```python
from build123d import *

# Parameters (mm, degrees)
ESQUISSE1_W                                    = 32
ESQUISSE1_H                                    = 18
BOSS_EXTRU_1_DEPTH                             = 2
ESQUISSE2_W                                    = 19
ESQUISSE2_H                                    = 14
BOSS_EXTRU_2_DEPTH                             = 1.4
FRAISAGE_POUR_VIS_T_TE_FRAIS_E_M21_D           = 2.6
FRAISAGE_POUR_VIS_T_TE_FRAIS_E_M21_CSINK_D     = 4.4
FRAISAGE_POUR_VIS_T_TE_FRAIS_E_M21_CSINK_ANGLE = 90
ESQUISSE6_W                                    = 15.8
ESQUISSE6_H                                    = 2
BOSS_EXTRU_3_DEPTH                             = 1.4
ESQUISSE7_W                                    = 19.2
ESQUISSE7_H                                    = 1.2
BOSS_EXTRU_4_DEPTH                             = 3.4
CONG_7_R                                       = 1


with BuildPart() as part:
    # Esquisse1 → Boss.-Extru.1 (new body)
    with BuildSketch(Plane.XY):
        Rectangle(ESQUISSE1_W, ESQUISSE1_H)
    extrude(amount=BOSS_EXTRU_1_DEPTH)

    # Esquisse2 → Boss.-Extru.2 (add)
    with BuildSketch(Plane(origin=(0, 0, 0), x_dir=(-1, 0, 0), z_dir=(0, 0, -1))):
        Rectangle(ESQUISSE2_W, ESQUISSE2_H)
    extrude(amount=BOSS_EXTRU_2_DEPTH)

    # Fraisage pour vis à tête fraisée M21 (through all)
    with Locations(Plane.XY.offset(2)):
        with Locations((-13, 0)):
            fraisage_pour_vis_t_te_frais_e_m21 = CounterSinkHole(FRAISAGE_POUR_VIS_T_TE_FRAIS_E_M21_D / 2, FRAISAGE_POUR_VIS_T_TE_FRAIS_E_M21_CSINK_D / 2, counter_sink_angle=FRAISAGE_POUR_VIS_T_TE_FRAIS_E_M21_CSINK_ANGLE)

    # Symétrie1: Fraisage pour vis à tête fraisée M21 across plane
    add(fraisage_pour_vis_t_te_frais_e_m21.mirror(Plane(origin=(0, 0, 0), x_dir=(0, 0, 1), z_dir=(1, 0, 0))), mode=Mode.SUBTRACT)

    # Esquisse6 → Boss.-Extru.3 (add)
    with BuildSketch(Plane(origin=(0, 0, 0), x_dir=(-1, 0, 0), z_dir=(0, 0, -1))):
        with Locations((0, 8)):
            Rectangle(ESQUISSE6_W, ESQUISSE6_H)
    extrude(amount=BOSS_EXTRU_3_DEPTH)

    # Esquisse7 → Boss.-Extru.4 (add)
    with BuildSketch(Plane.XY.offset(2)):
        with Locations((0, 6.4)):
            Rectangle(ESQUISSE7_W, ESQUISSE7_H)
    extrude(amount=-BOSS_EXTRU_4_DEPTH)

    # Congé7
    cong_7_edges = [part.edges().sort_by_distance(p)[0] for p in [
        (16, -9, 1),
        (-16, -9, 1),
    ]]
    fillet(cong_7_edges, radius=CONG_7_R)


solid = part.part
```
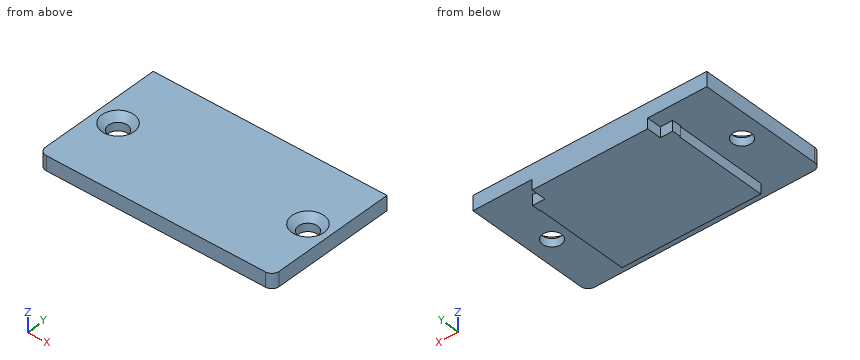
The listing builds one solid part. Answer for the finished solid, in the listing's coordinates (mm). Give positions to 0.01 mm unless a question says otherwise; leave off trailing zeros. Loops run counter-clockwise (first coordinate to the right, second up) from the corner with the lowest first, then second, coordinate; pieces in that order, holes last. Notation, with made-up numbers: (40, 44) - (68, 44) arc R22 cw to (68, 68) - close; hole circle Ø2 at (21.5, 46). An arc over 180 degrees is marked (long way). Return JSON: item names as keys, results as strings. Group by question number.
1. Find section B-B (z = 0.55). Write down the section's boundary in (x, y), then the cut area to 3 significant figures.
2. Find section C-C (x = -13). Write down the section's boundary in (y, z), then the cut area to 3 significant figures.
3. Straight lines are drawn through the part: line 1 (X direction, y = 0, z = 0.6); line 2 (Y direction, x = -13, z = 0.4); line 3 (X direction, y = 3.25, z = -0.95). For each, find the intervals that lie inside material, in ascending order. Write a range as [from, to].
4. Find section A-A (y = 0). Write down the section's boundary in (x, z), then the cut area to 3 significant figures.
5. Find section D-D (z = -0.8). Write down the section's boundary in (x, y), then the cut area to 3 significant figures.
6. Given pin 1 Ø1.1 at (y, z) = (-1, -1) entering from +X; pin 2 Ø1.1 at (y, z) = (7.5, -1) entering from -X; pin 3 Ø1.5 at (y, z) = (8.5, -1) entering from +X; pin 4 Ø1.6 at (x, y) = (13, 0) entering from +Z, each flat-ended and moving along its own axis, determine where each tip first touches the part or whether it passes through.
Verdict:
{
 "1": {"outline": "(-16, -8) arc R1 ccw to (-15, -9) - (15, -9) arc R1 ccw to (16, -8) - (16, 9) - (-16, 9) - close; hole circle Ø2.6 at (-13, 0); hole circle Ø2.6 at (13, 0)", "area": "565 mm^2"},
 "2": {"outline": "(-9, 0) - (-1.3, 0) - (-1.3, 1.1) - (-2.2, 2) - (-9, 2) - close; (1.3, 0) - (9, 0) - (9, 2) - (2.2, 2) - (1.3, 1.1) - close", "area": "30.0 mm^2"},
 "3": {"line 1": "x = [-16, -14.3], [-11.7, 11.7], [14.3, 16]", "line 2": "y = [-9, -1.3], [1.3, 9]", "line 3": "x = [-9.5, 9.5]"},
 "4": {"outline": "(-16, 0) - (-14.3, 0) - (-14.3, 1.1) - (-15.2, 2) - (-16, 2) - close; (-11.7, 0) - (-9.5, 0) - (-9.5, -1.4) - (9.5, -1.4) - (9.5, 0) - (11.7, 0) - (11.7, 1.1) - (10.8, 2) - (-10.8, 2) - (-11.7, 1.1) - close; (14.3, 0) - (16, 0) - (16, 2) - (15.2, 2) - (14.3, 1.1) - close", "area": "78.6 mm^2"},
 "5": {"outline": "(-9.6, 5.8) - (-9.5, 5.8) - (-9.5, -7) - (9.5, -7) - (9.5, 5.8) - (9.6, 5.8) - (9.6, 7) - (7.9, 7) - (7.9, 9) - (-7.9, 9) - (-7.9, 7) - (-9.6, 7) - close", "area": "298 mm^2"},
 "6": {"pin 1": "stops at x = 9.5", "pin 2": "stops at x = -9.6", "pin 3": "stops at x = 7.9", "pin 4": "passes through"}
}
